Can you work these out from the model? Positions are in its coordinate system, mm. A direction names the side the tool comes from. Round coordinates to 2 decimals unless told otherwise and drop trailing zeros. Order: outer loops, then holes, each group sorted by start corner. A loop starts at its lowest first (then second) coordinate and runs counter-clockwise, first axis right, second up.
from build123d import *

# Parameters (mm, degrees)
SKETCH1_R                = 6.35
SKETCH1_R_2              = 5.842
BOSS_EXTRUDE1_DEPTH      = 3.96748
BOSS_EXTRUDE2_DEPTH      = 4.36499
BOSS_EXTRUDE2_DEPTH_BACK = 0.39751
SKETCH1_3_R              = 4.572
SKETCH1_3_R_2            = 3.96875
BOSS_EXTRUDE3_START      = 0.41148
SKETCH1_4_R              = 5.842
SKETCH1_4_R_2            = 4.572
BOSS_EXTRUDE3_DEPTH      = 3.14452


with BuildPart() as part:
    # Sketch1 → Boss-Extrude1 (new body)
    with BuildSketch(Plane.XY):
        Circle(SKETCH1_R)
        Circle(SKETCH1_R_2, mode=Mode.SUBTRACT)
    extrude(amount=BOSS_EXTRUDE1_DEPTH)



with BuildPart() as body_2:
    # Sketch1<3> → Boss-Extrude2 (new, two sides: drawn at the far end of the back side and taken through both)
    with BuildSketch(Plane.XY.offset(-BOSS_EXTRUDE2_DEPTH_BACK)):
        Circle(SKETCH1_3_R)
        Circle(SKETCH1_3_R_2, mode=Mode.SUBTRACT)
    extrude(amount=BOSS_EXTRUDE2_DEPTH + BOSS_EXTRUDE2_DEPTH_BACK)


with BuildPart() as part_1:
    add(part.part)

    add(body_2.part)  # Boss-Extrude3 merges body 2
    # Sketch1<4> → Boss-Extrude3 (add)
    with BuildSketch(Plane.XY.offset(BOSS_EXTRUDE3_START)):
        Circle(SKETCH1_4_R)
        Circle(SKETCH1_4_R_2, mode=Mode.SUBTRACT)
    extrude(amount=BOSS_EXTRUDE3_DEPTH)


solid = part_1.part
(1) On a 3-axis mill with a long thin cutter (end or side, diameter ignored), from which of +Z, -Z, +X, -X, +Y, -Y can I reach the whole of each face in a straight line? I mean faces 4 (the face through (3, -4, 0.411)), 5 (the face through (-0.991, -4.463, 3.955)), 6 (the face through (-1, 4, -0.398)). Say none if no direction works.
(2) I want a section at D-D, the plane y = -5.5. List the corners of the cut face in (x, z) for me, plus the area to 3 significant figures.
(3) If we mould it in two halves opening along Y, with no side actions, what happens to faces 1 (the face through (-1, 4, 4.365)), 2 (the face through (-1.38, -6.2, 1.96)), 3 (the face through (-1.266, -5.703, 0.203))? For each: pulls with the +Y half, pulls with the -Y half, needs draft (parallel to the pull), parting line crosses it, or undercut.
(4) I want a section at C-C, the plane z = 0.15. List the corners of the cut face in (x, y) for me.
(5) I'm going to push flat-ended pins straight in: pin 1 Ø7 at (x, y) = (0, 0) entering from +Z; pin 2 Ø1 at (y, z) = (3, 2) entering from +X. Where does each tip first touch, or does it pass through?
(6) Please list where these lines run through material, in increasing order: probe 1 along Y at (x, z) = (0, 0.3); probe 2 along Y at (x, z) = (0, 2.7); probe 3 along Z at (x, y) = (5.5, -1.5).
(7) I want a section at A-A, the plane y = 0. List the corners of the cut face in (x, z) for me, plus the area to 3 significant figures.
Ans:
1. face 4: -Z
1. face 5: +Z
1. face 6: -Z, +X, -X, +Y, -Y
2. outline: (-3.17, 0) - (-1.97, 0) - (-1.97, 0.41) - (1.97, 0.41) - (1.97, 0) - (3.17, 0) - (3.17, 3.97) - (1.97, 3.97) - (1.97, 3.56) - (-1.97, 3.56) - (-1.97, 3.97) - (-3.17, 3.97) - close
2. area: 21.9 mm2
3. face 1: needs draft
3. face 2: parting line crosses it
3. face 3: undercut
4. outline: circle Ø12.7 at (0, 0); circle Ø9.14 at (0, 0); hole circle Ø11.68 at (0, 0); hole circle Ø7.94 at (0, 0)
5. pin 1: passes through
5. pin 2: stops at x = 5.84
6. probe 1: y = -6.35 to -5.84, -4.57 to -3.97, 3.97 to 4.57, 5.84 to 6.35
6. probe 2: y = -6.35 to -3.97, 3.97 to 6.35
6. probe 3: z = 0.41 to 3.56
7. outline: (-6.35, 0) - (-5.84, 0) - (-5.84, 0.41) - (-4.57, 0.41) - (-4.57, -0.4) - (-3.97, -0.4) - (-3.97, 4.36) - (-4.57, 4.36) - (-4.57, 3.56) - (-5.84, 3.56) - (-5.84, 3.97) - (-6.35, 3.97) - close; (3.97, -0.4) - (4.57, -0.4) - (4.57, 0.41) - (5.84, 0.41) - (5.84, 0) - (6.35, 0) - (6.35, 3.97) - (5.84, 3.97) - (5.84, 3.56) - (4.57, 3.56) - (4.57, 4.36) - (3.97, 4.36) - close
7. area: 17.8 mm2
